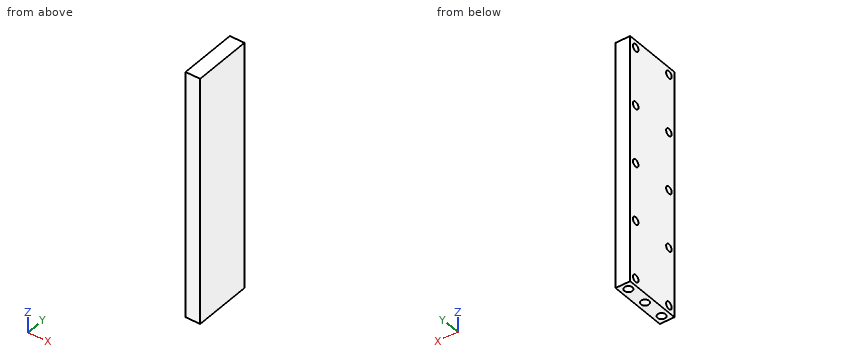
from build123d import *

# Parameters (mm, degrees)
CROQUIS1_W              = 170
CROQUIS1_H              = 40
SALIENTE_EXTRUIR1_DEPTH = 5
CROQUIS2_R              = 2.5
CORTAR_EXTRUIR1_DEPTH   = 5
CROQUIS3_R              = 2.748332181
CORTAR_EXTRUIR2_DEPTH   = 5


with BuildPart() as part:
    # Croquis1 → Saliente-Extruir1 (new, symmetric)
    with BuildSketch(Plane(origin=(0, 0, 0), x_dir=(0, 0, -1), z_dir=(1, 0, 0))):
        Rectangle(CROQUIS1_W, CROQUIS1_H)
    extrude(amount=SALIENTE_EXTRUIR1_DEPTH, both=True)

    # Croquis2 → Cortar-Extruir1 (cut)
    with BuildSketch(Plane(origin=(0, 0, 0), x_dir=(0, 0, -1), z_dir=(1, 0, 0))):
        with Locations((-80, 15)):
            Circle(CROQUIS2_R)
        with Locations((-40, 15)):
            Circle(CROQUIS2_R)
        with Locations((0, 15)):
            Circle(CROQUIS2_R)
        with Locations((40, 15)):
            Circle(CROQUIS2_R)
        with Locations((80, 15)):
            Circle(CROQUIS2_R)
        with Locations(Location((80, -15, 0), (0, 0, 180))):
            Circle(CROQUIS2_R)
        with Locations(Location((40, -15, 0), (0, 0, 180))):
            Circle(CROQUIS2_R)
        with Locations(Location((0, -15, 0), (0, 0, 180))):
            Circle(CROQUIS2_R)
        with Locations(Location((-40, -15, 0), (0, 0, 180))):
            Circle(CROQUIS2_R)
        with Locations(Location((-80, -15, 0), (0, 0, 180))):
            Circle(CROQUIS2_R)
    extrude(amount=-CORTAR_EXTRUIR1_DEPTH, mode=Mode.SUBTRACT)

    # Croquis3 → Cortar-Extruir2 (cut)
    with BuildSketch(Plane(origin=(0, 0, -85), x_dir=(-1, 0, 0), z_dir=(0, 0, -1))):
        with Locations((0, 15)):
            Circle(CROQUIS3_R)
        with Locations(Location((0, -15, 0), (0, 0, 294.543993406))):
            Circle(CROQUIS3_R)
        Circle(CROQUIS3_R)
    extrude(amount=-CORTAR_EXTRUIR2_DEPTH, mode=Mode.SUBTRACT)


solid = part.part
Read the model definition and answer for the solid it produces. Units are mm, in the model's axes. Round coordinates to 2 decimals unless told otherwise and drop trailing zeros. Loops run counter-clockwise (first coordinate to the right, second up) from the corner with the lowest first, then second, coordinate; pieces in that order, holes last.
Q1. Each of these flat-tipped pins is pushed along its axis until it touches: pin 1 (1.2 mm diameter, centred on x = 2, y = -14.5, fed in from -Z); pin 2 (1.5 mm diameter, centred on y = -15.5, z = 40.5, fed in from -X). Where does it stop, or does it pass through?
Q2. Consider probe 1 along Y at (x, z) = (-3.35, 0); probe 2 along Z at (x, y) = (-1.35, -15); probe 3 along Y at (x, z) = (0, -83.55). Determine where each line is inside the solid, lowest interval first.
Q3. Section A-A on y = -15 is taken. Write down the section's boundary in (x, z).
Q4. Section B-B on z = 40 is taken. Write down the section's boundary in (x, y).
Output:
1. pin 1: stops at z = -80
1. pin 2: stops at x = 0
2. probe 1: y = -20 to -17.5, -12.5 to 12.5, 17.5 to 20
2. probe 2: z = -77.5 to -42.5, -37.5 to -2.5, 2.5 to 37.5, 42.5 to 77.5, 82.5 to 85
2. probe 3: y = -20 to -17.75, -12.25 to -2.75, 2.75 to 12.25, 17.75 to 20
3. outline: (-5, -85) - (-2.75, -85) - (-2.75, -82.5) - (-5, -82.5) - close; (-5, -77.5) - (0, -77.5) - (0, -80) - (2.75, -80) - (2.75, -85) - (5, -85) - (5, 85) - (-5, 85) - (-5, 82.5) - (0, 82.5) - (0, 77.5) - (-5, 77.5) - (-5, 42.5) - (0, 42.5) - (0, 37.5) - (-5, 37.5) - (-5, 2.5) - (0, 2.5) - (0, -2.5) - (-5, -2.5) - (-5, -37.5) - (0, -37.5) - (0, -42.5) - (-5, -42.5) - close
4. outline: (-5, -20) - (5, -20) - (5, 20) - (-5, 20) - (-5, 17.5) - (0, 17.5) - (0, 12.5) - (-5, 12.5) - (-5, -12.5) - (0, -12.5) - (0, -17.5) - (-5, -17.5) - close
